Input: dimensioned drawing with shaded views. Units: mm. Origin: part minimum x, y, z. Give positions to 0.01 mm unless a question says otherwise; leave off trailing zeros. Loops run counter-clockwise (first coordinate to the right, second up) from the corner with the lowest first, then second, coordinate; pieces in that order, holes last. Notation, with made-up numbers: (81, 54) -> (136, 54) arc R23 cw to (136, 83) -> close; hole circle Ø3 at (21, 19). An arc over 180 degrees is marked (long way). Answer in a Markdown table with one row per item. Add a question column.
1) First-contact query: P1, Ø1.6, axis at y = 1.5, z = 129, coming from the +X side; P2, Ø1, axis at x = 1.5, y = 2.5, coming from the +Z side; P3, Ø1.6, axis at x = 1, y = 2, coming from the -Z side. Flat tips, straight axial feed; report the tip coordinate or a pass-through.
2) Section query A-A (z = 129). Return the cut outline in (x, y) (3 decimals).
3) Line query: line 1 (X direction, y = 0.3, z = 19) (3 decimals). Output: solid intervals per line, ascending. Write a range as from..to.
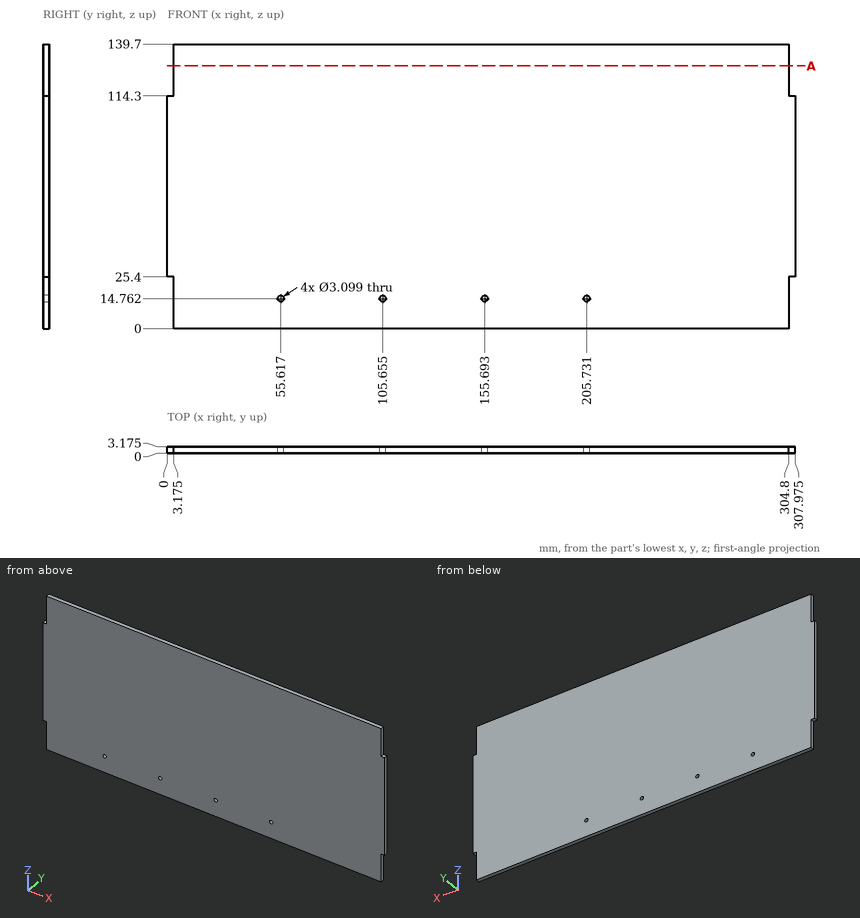
Evaluation:
| question | item | result |
|---|---|---|
| 1 | P1 | x = 304.8 |
| 1 | P2 | z = 114.3 |
| 1 | P3 | z = 25.4 |
| 2 | outline | (3.175, 0) -> (304.8, 0) -> (304.8, 3.175) -> (3.175, 3.175) -> close |
| 3 | line 1 | 3.175..304.8 |
